Study the drawing (mm; zero at the part's minimum x, y, z) and answer. A direction names the side the tool comes from. Coordinates: 2 decimals unless noted, no trailing zeros. Order: outer loops, then holes, each group sorted by start corner. A loop starts at its lowest first (then second) coordinate and runs counter-clockwise, first axis right, second up. Notation, with made-up numbers: (-21, 76) -> (-11, 76) arc R33 cw to (-11, 107) -> close; hole circle Ø4 at (4, -20.5). An arc over 180 degrees is marked (long way). Write each question's results on one line, items separated by ' | '. Start each with the question number.
(1) Straight lines are drawn through the part: L1, parallel to Z at x = 6, y = 2.5; L2, parallel to X at y = 1, z = 8.75; L3, parallel to X at y = 3.3, z = 13.75. For each, find the intervals that lie inside material, in ascending order.
(2) The part is cut by section B-B, the plane z = 11. Give the vertices of the cut face in (x, y), then the cut area to 3 significant figures.
(3) Determine the mould class of the marked faces 3, 4 and 5 for opening direction Z: +Z half, -Z half, draft (parallel to the pull), parting line (faces both ways), or undercut.
(4) A tool of negligible diameter and unlimited length cuts with its end or side. For the marked faces 1 and 2, from which of +Z, -Z, +X, -X, +Y, -Y can it reach the whole face along a straight path? Write none if from no direction.
(5) The part is cut by section C-C, the plane x = 6. Give the vertices of the cut face in (y, z), then the cut area to 3 significant figures.
(6) The part is cut by section A-A, the plane x = 19.4. Give the vertices of the cut face in (y, z).
(7) The part is cut by section D-D, the plane y = 1.4. Give the vertices of the cut face in (x, z), then the cut area to 3 significant figures.
(8) Given pin 1 (2 mm diameter, centred on x = 6, z = 14.686, fed in from +Y), flat-ended and moving along its own axis, determine where the tip first touches the part or whether it passes through.
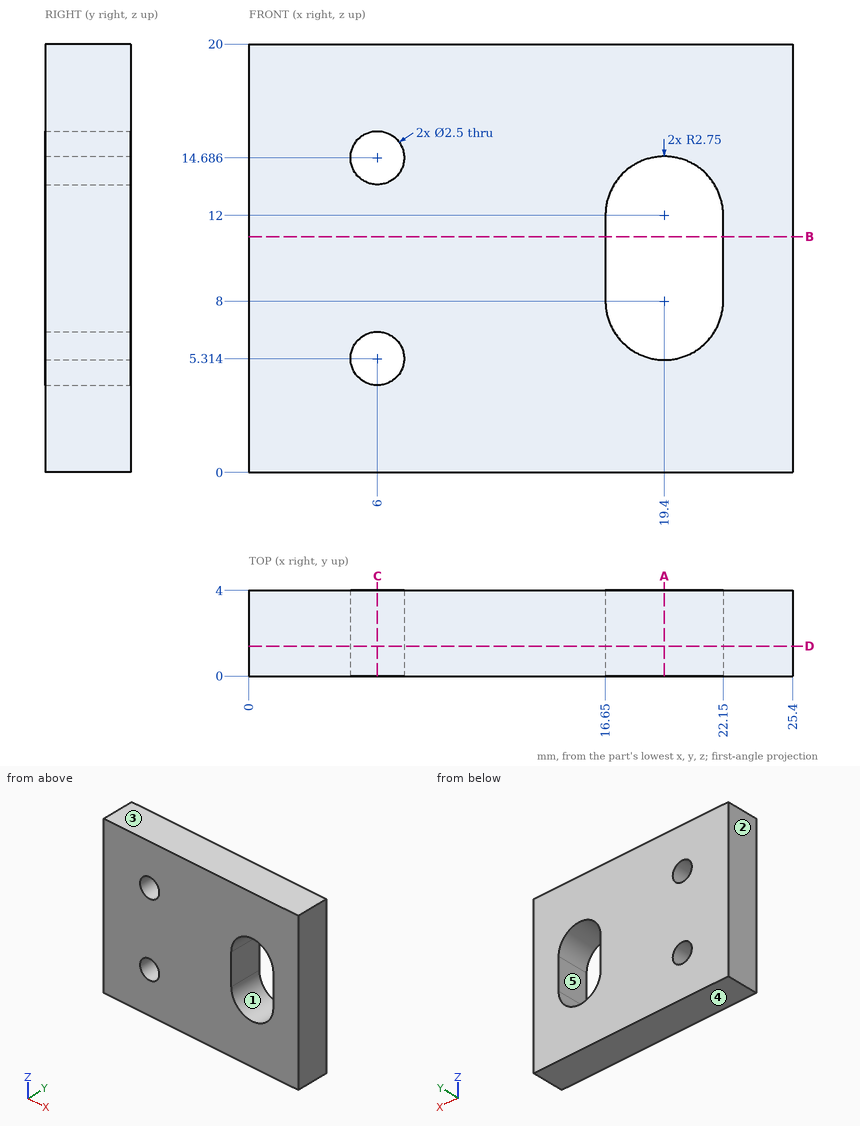
Established:
1) L1: z = 0 to 4.06, 6.56 to 13.44, 15.94 to 20 | L2: x = 0 to 16.65, 22.15 to 25.4 | L3: x = 0 to 5.17, 6.83 to 17.28, 21.52 to 25.4
2) outline: (0, 0) -> (16.65, 0) -> (16.65, 4) -> (0, 4) -> close; (22.15, 0) -> (25.4, 0) -> (25.4, 4) -> (22.15, 4) -> close | area: 79.6 mm^2
3) face 3: +Z half | face 4: -Z half | face 5: undercut
4) face 1: +Y, -Y | face 2: +Z, -Z, -X, +Y, -Y
5) outline: (0, 0) -> (4, 0) -> (4, 4.06) -> (0, 4.06) -> close; (0, 6.56) -> (4, 6.56) -> (4, 13.44) -> (0, 13.44) -> close; (0, 15.94) -> (4, 15.94) -> (4, 20) -> (0, 20) -> close | area: 60.0 mm^2
6) outline: (0, 0) -> (4, 0) -> (4, 5.25) -> (0, 5.25) -> close; (0, 14.75) -> (4, 14.75) -> (4, 20) -> (0, 20) -> close
7) outline: (0, 0) -> (25.4, 0) -> (25.4, 20) -> (0, 20) -> close; hole circle Ø2.5 at (6, 5.31); hole circle Ø2.5 at (6, 14.69); hole (16.65, 8) arc R2.75 ccw to (22.15, 8) -> (22.15, 12) arc R2.75 ccw to (16.65, 12) -> close | area: 452 mm^2
8) pin 1: passes through
